Autodesk Inventor part; units mm, degrees
ref_plane "YZ Plane" through (0, 0, 0) normal (1, 0, 0) x (0, 1, 0)
ref_plane "XZ Plane" through (0, 0, 0) normal (0, 1, 0) x (-1, 0, 0)
ref_plane "XY Plane" through (0, 0, 0) normal (0, 0, 1) x (1, 0, 0)
sketch "Эскиз1" plane through (0, 0, 0) normal (0, 0, 1) x (1, 0, 0)
  line L0 (0, 0) -> (0, 5)
  line L1 (0, 0) -> (-7, 0)
  line L2 (-7, 0) -> (0, 5)
  line L3 (0, 5) -> (4, 5)
  line L4 (4, 5) -> (4, 0)
  line L5 (4, 0) -> (0, 0)
  dimension "d0" = 5
  dimension "d1" = 7
  dimension "d2" = 4
extrude "Выдавливание1" add sketch "Эскиз1" along normal blind 3
sketch "Эскиз2" plane through (0, 0, 3) normal (0, 0, 1) x (1, 0, 0)
  line L0 (-7, 0) -> (4, 0)
  line L1 (-7, 0) -> (-11, 0)
  line L2 (4, 5) -> (0, 5)
  line L3 (0, 5) -> (0, 9)
  line L4 (0, 9) -> (-11, 0)
  line L5 (4, 5) -> (4, 9)
  line L6 (4, 9) -> (0, 9)
  line L7 (4, 0) -> (4, 5)
  line L8 (4, 5) -> (4, 0)
  line L9 (4, 0) -> (-7, 0)
  point P0 (0, 0)
  dimension "d5" = 4
  dimension "d6" = 4
extrude "Выдавливание2" add sketch "Эскиз2" along normal blind 2
sketch "Эскиз3" plane through (0, 0, 0) normal (0, 0, -1) x (-1, 0, 0)
  line L0 (-4, 0) -> (-4, 5)
  line L1 (-4, 0) -> (-4, 3)
  line L2 (-4, 3) -> (2.8, 3)
  line L3 (0, 5) -> (7, 0)
  line L4 (7, 0) -> (-4, 0)
  line L5 (2.8, 3) -> (7, 0)
  line L6 (7, 0) -> (-4, 0)
  line L7 (2.8, 3) -> (2.8, 0)
  point P0 (0, 0)
  dimension "d9" = 3
extrude "Выдавливание3" add sketch "Эскиз3" along normal blind 5 contours L0 L2 L7 L4
fillet "Сопряжение1" radius 1 10 edges at (4, 3, -2.5) (4, 0, 0) (-2.8, 0, -2.5) (-2.8, 3, -2.5) (0, 5, 1.5) (0, 9, 4) (0.6, 3, -5) (4, 1.5, -5) (0.6, 0, -5) (-2.8, 1.5, -5)
properties part number "разделитель"
Verification items for the finished model (mm, model axes). A direction names the side the tool comes from. Round coordinates to 2 decimals unless told otherwise and drop trailing zeros. Order: outer loops, then holes, each group sorted by start corner. A loop starts at its lowest first (then second) coordinate and runs counter-clockwise, first axis right, second up. Notation, with made-up numbers: (45.5, -7.5) -> (51.5, -7.5) arc R13 ccw to (51.5, 15.5) -> close; hole circle Ø4 at (17.5, -27.5). An arc over 180 degrees is marked (long way). Put each result on its own line as item: value. Start each with the question number.
(1) Section check B-B (z = -2.75). Enter the section's corners in (x, y).
(2) Material ranges on line 1 along Z through (x, y) = (-4.5, 1.5); line 2 along Z through (x, y) = (-4.5, 2), recorded low to high.
(3) Section check C-C (x = 1.5). Enter the section's corners in (y, z), then the cut area to 3 significant figures.
(4) Depth check by flat-ended pin: pin 1 Ø3 at (x, z) = (0, -3) entering from +Y. Enter the tip coordinate at first touch or a pass-through.
(5) Tool access check on faces 1 (the face through (-2.499, 0.285, -2.028)), 2 (the face through (-2, 5, 3)), 3 (the face through (3.699, 2.715, -2.028)), 4 (the face through (1, 3, -2)). Record the directions out of +Z, -Z, +X, -X, +Y, -Y that give a thin tool (end or side, any length) a straight path to the whole face; none if there is none.
(6) Section check A-A (y = 4.5). Enter the section's corners in (x, z).
(7) Section check D-D (x = 3.25). Enter the section's corners in (y, z).
Completed:
1. outline: (-2.8, 1) arc R1 ccw to (-1.8, 0) -> (3, 0) arc R1 ccw to (4, 1) -> (4, 2) arc R1 ccw to (3, 3) -> (-1.8, 3) arc R1 ccw to (-2.8, 2) -> close
2. line 1: z = 0 to 5
2. line 2: z = 3 to 5
3. outline: (0, -4) arc R1 ccw to (1, -5) -> (2, -5) arc R1 ccw to (3, -4) -> (3, 0) -> (5, 0) -> (5, 3) -> (9, 3) -> (9, 5) -> (0, 5) -> close
3. area: 47.6 mm2
4. pin 1: stops at y = 3
5. face 1: -Z, -X, -Y
5. face 2: -Z, -X, +Y
5. face 3: -Z, +X, +Y
5. face 4: -Z, +X, -X, +Y
6. outline: (-5.5, 3) -> (-0.7, 3) -> (-0.7, 0) -> (4, 0) -> (4, 5) -> (-5.5, 5) -> close
7. outline: (0.03, -4) arc R0.97 ccw to (1, -4.97) -> (2, -4.97) arc R0.97 ccw to (2.97, -4) -> (2.97, 0) -> (5, 0) -> (5, 3) -> (9, 3) -> (9, 5) -> (0.03, 5) -> close
